Verification items for the finished model (mm, model axes). Round coordinates to 2 decimals unless told otherwise and drop trailing zeros. Loops run counter-clockwise (first coordinate to the right, second up) from the corner with the lowest first, then second, coordinate; pieces in that order, holes last. Notation, with made-up numbers: M 39.25,64.25 L 43.25,64.25 A15 cw 43.25,74.25 Z; hole C -9,20.5 d7. An arc over 180 degrees is marked long. One line per item, written item: value.
from build123d import *

# Parameters (mm, degrees)
SKETCH1_W           = 85.1662
SKETCH1_H           = 22.225
BOSS_EXTRUDE1_DEPTH = 1.5875
CUT_EXTRUDE1_REACH  = 3.587
SKETCH2_R           = 2.667


with BuildPart() as part:
    # Sketch1 → Boss-Extrude1 (new body)
    with BuildSketch(Plane(origin=(0, 0, 0), x_dir=(1, 0, 0), z_dir=(0, 1, 0))):
        with Locations((42.5831, 11.1125)):
            Rectangle(SKETCH1_W, SKETCH1_H)
    extrude(amount=BOSS_EXTRUDE1_DEPTH)

    # Sketch2 → Cut-Extrude1 (cut, up to next)
    with BuildSketch(Plane.XZ, mode=Mode.PRIVATE) as cut_extrude1_sk1:
        with Locations((4.7625, -7.112)):
            Circle(SKETCH2_R)
    cut_extrude1_tool1 = extrude(cut_extrude1_sk1.sketch, amount=-CUT_EXTRUDE1_REACH, mode=Mode.PRIVATE) & part.part
    add(cut_extrude1_tool1.solids().sort_by_distance((4.7625, 0, -7.112))[0], mode=Mode.SUBTRACT)
    # Sketch2 → Cut-Extrude1 (cut, up to next)
    with BuildSketch(Plane.XZ, mode=Mode.PRIVATE) as cut_extrude1_sk2:
        with Locations((12.7, -14.478)):
            Circle(SKETCH2_R)
    cut_extrude1_tool2 = extrude(cut_extrude1_sk2.sketch, amount=-CUT_EXTRUDE1_REACH, mode=Mode.PRIVATE) & part.part
    add(cut_extrude1_tool2.solids().sort_by_distance((12.7, 0, -14.478))[0], mode=Mode.SUBTRACT)
    # Sketch2 → Cut-Extrude1 (cut, up to next)
    with BuildSketch(Plane.XZ, mode=Mode.PRIVATE) as cut_extrude1_sk3:
        with Locations((72.4662, -7.112)):
            Circle(SKETCH2_R)
    cut_extrude1_tool3 = extrude(cut_extrude1_sk3.sketch, amount=-CUT_EXTRUDE1_REACH, mode=Mode.PRIVATE) & part.part
    add(cut_extrude1_tool3.solids().sort_by_distance((72.4662, 0, -7.112))[0], mode=Mode.SUBTRACT)
    # Sketch2 → Cut-Extrude1 (cut, up to next)
    with BuildSketch(Plane.XZ, mode=Mode.PRIVATE) as cut_extrude1_sk4:
        with Locations((80.4037, -14.478)):
            Circle(SKETCH2_R)
    cut_extrude1_tool4 = extrude(cut_extrude1_sk4.sketch, amount=-CUT_EXTRUDE1_REACH, mode=Mode.PRIVATE) & part.part
    add(cut_extrude1_tool4.solids().sort_by_distance((80.4037, 0, -14.478))[0], mode=Mode.SUBTRACT)


solid = part.part
(1) Mould release check, pull along X, two halves, no side actions. Record for faces 1 (the face through (42, 0, -11)), 2 (the face through (0, 1, -11)), 3 (the face through (15.164, 0.783, -15.499)): +X half, -X half, draft (parallel to the pull), parting line (faces both ways), or undercut.
Completed:
face 1: draft
face 2: -X half
face 3: undercut
(2) Sectioned sample at B-B on y = 1.3. Enter the section's corners in (x, z) (1 decimal), and give its area (3 significant figures).
Completed:
outline: M 0,-22.2 L 85.2,-22.2 L 85.2,0 L 0,0 Z; hole C 4.8,-7.1 d5.3; hole C 12.7,-14.5 d5.3; hole C 72.5,-7.1 d5.3; hole C 80.4,-14.5 d5.3
area: 1,800 mm^2
(3) Sectioned sample at C-C on z = -13.75. Enter the section's corners in (x, y).
Completed:
outline: M 0,0 L 10.13,0 L 10.13,1.59 L 0,1.59 Z; M 15.27,0 L 77.84,0 L 77.84,1.59 L 15.27,1.59 Z; M 82.97,0 L 85.17,0 L 85.17,1.59 L 82.97,1.59 Z
(4) Sectioned sample at A-A on x = 12.7. Enter the section's corners in (y, z) (1 decimal), and give its area (3 significant figures).
Completed:
outline: M 0,-22.2 L 1.6,-22.2 L 1.6,-17.1 L 0,-17.1 Z; M 0,-11.8 L 1.6,-11.8 L 1.6,0 L 0,0 Z
area: 26.8 mm^2
(5) Thickness scan on L1, parallel to X at y = 1.55, z = -14.5; L2, parallel to Z at x = 12.7, y = 0.65 (3 decimals); L3, parallel to X at y = 0.5, z = -9.5. Record the ranges inside material, lowest first. Write a range as from..to.
Completed:
L1: x = 0..10.03, 15.37..77.74, 83.07..85.17
L2: z = -22.225..-17.145, -11.811..0
L3: x = 0..3.57, 5.95..71.28, 73.65..85.17
(6) Sectioned sample at D-D on z = -6.25. Enter the section's corners in (x, y), and give its area (3 significant figures).
Completed:
outline: M 0,0 L 2.24,0 L 2.24,1.59 L 0,1.59 Z; M 7.29,0 L 69.94,0 L 69.94,1.59 L 7.29,1.59 Z; M 74.99,0 L 85.17,0 L 85.17,1.59 L 74.99,1.59 Z
area: 119 mm^2
